```python
from build123d import *

# Parameters (mm, degrees)
F0_W     = 430
F0_H     = 130
F1_DEPTH = 22
F2_W     = 22
F2_H     = 22
F2_H_2   = 20
F3_DEPTH = 25


with BuildPart() as f1:
    # F0 (on Front) → F1 (new body)
    with BuildSketch(Plane.XZ):
        with Locations((215, 65)):
            Rectangle(F0_W, F0_H)
    extrude(amount=F1_DEPTH)

    # F2 (on face) → F3 (cut)
    with BuildSketch(Plane.XZ.offset(22)):
        with Locations((11, 33)):
            Rectangle(F2_W, F2_H)
        with Locations((11, 77)):
            Rectangle(F2_W, F2_H)
        with Locations((419, 77)):
            Rectangle(F2_W, F2_H)
        with Locations((419, 33)):
            Rectangle(F2_W, F2_H)
        with Locations((11, 120)):
            Rectangle(F2_W, F2_H_2)
        with Locations((419, 120)):
            Rectangle(F2_W, F2_H_2)
    extrude(amount=-F3_DEPTH, mode=Mode.SUBTRACT)


solid = f1.part
```
Geometry check sheet. Reference: the model listing, model coordinates, mm. A direction names the side the tool comes from. Give positions to 0.01 mm unless a question says otherwise; leave off trailing zeros. Loops run counter-clockwise (first coordinate to the right, second up) from the corner with the lowest first, then second, coordinate; pieces in that order, holes last. Notation, with made-up numbers: M 28,55 L 79,55 A27 cw 79,79 Z; hole C 20.5,-33.75 d4. An arc over 180 degrees is marked long. Answer as CSV lines item,"result".
Item 1: Cross-section at B-B on z = 77. Record the cut outline in (x, y).
Values:
outline,"M 22,-22 L 408,-22 L 408,0 L 22,0 Z"
Item 2: Depth check by flat-ended pin: P1, Ø6.5, axis at y = -7, z = 34, coming from the +X side; P2, Ø11, axis at x = 419.5, y = -12, coming from the +Z side; P3, Ø6, axis at y = -9, z = 124, coming from the -X side. Enter the tip coordinate at first touch or a pass-through.
Values:
P1,"stops at x = 408"
P2,"stops at z = 110"
P3,"stops at x = 22"
Item 3: Material ranges on line 1 (X direction, y = -10.75, z = 111), recorded low to high.
Values:
line 1,"x = 22 to 408"
Item 4: Cross-section at A-A on y = -5. Record the cut outline in (x, z).
Values:
outline,"M 0,0 L 430,0 L 430,22 L 408,22 L 408,44 L 430,44 L 430,66 L 408,66 L 408,88 L 430,88 L 430,110 L 408,110 L 408,130 L 22,130 L 22,110 L 0,110 L 0,88 L 22,88 L 22,66 L 0,66 L 0,44 L 22,44 L 22,22 L 0,22 Z"
Item 5: Access from +Z, -Z, +X, -X, +Y, -Y to the whole of each face (thin tool, end or side, straight path). Record for faces 1 (the flat face through (11, -11, 66)), 2 (the flat face through (408, -11, 120)), 3 (the flat face through (408, -11, 33)), 4 (the flat face through (22, -11, 120)), 5 (the flat face through (0, -11, 99)).
Values:
face 1,"-X, +Y, -Y"
face 2,"+Z, +X, +Y, -Y"
face 3,"+X, +Y, -Y"
face 4,"+Z, -X, +Y, -Y"
face 5,"+Z, -Z, -X, +Y, -Y"
